Autodesk Inventor part; units mm, degrees
ref_plane "Work Plane1" through (60.325, 6.35, 63.5) normal (1, 0, 0) x (0, 0, -1)
ref_plane "Work Plane2" through (60.325, 6.35, -26.9875) normal (1, 0, 0) x (0, 0, -1)
ref_plane "YZ Plane" through (0, 0, 0) normal (1, 0, 0) x (0, 1, 0)
sketch "Sketch1" plane through (0, 0, 0) normal (0, 1, 0) x (-1, 0, 0)
  line L0 (0, -88.9) -> (0, 88.9)
  line L1 (-102.235, 0) -> (124.46, 0)
  line L2 (50.8, 44.45) -> (-50.8, 44.45)
  line L3 (-50.8, -44.45) -> (50.8, -44.45)
  line L4 (50.8, -44.45) -> (50.8, 44.45)
  line L5 (76.2, 63.5) -> (-69.85, 63.5)
  line L6 (-69.85, -63.5) -> (76.2, -63.5)
  line L7 (76.2, -63.5) -> (76.2, 63.5)
  line L8 (-50.8, 26.9875) -> (-69.85, 26.9875)
  line L9 (-69.85, -26.9875) -> (-50.8, -26.9875)
  line L10 (-50.8, 44.45) -> (-50.8, 26.9875)
  line L11 (-50.8, -26.9875) -> (-50.8, -44.45)
  line L12 (-69.85, 63.5) -> (-69.85, 26.9875)
  line L13 (-69.85, -26.9875) -> (-69.85, -63.5)
  line L14 (-53.975, 63.5) -> (-66.675, 63.5) construction
  line L15 (-66.675, 63.5) -> (-66.675, 26.9875) construction
  line L16 (-66.675, 26.9875) -> (-53.975, 26.9875) construction
  line L17 (-53.975, 26.9875) -> (-53.975, 63.5) construction
  line L18 (-53.975, -26.9875) -> (-66.675, -26.9875) construction
  line L19 (-66.675, -26.9875) -> (-66.675, -63.5) construction
  line L20 (-66.675, -63.5) -> (-53.975, -63.5) construction
  line L21 (-53.975, -63.5) -> (-53.975, -26.9875) construction
  line L22 (-60.325, 63.5) -> (-60.325, 26.9875) construction
  line L23 (-60.325, -26.9875) -> (-60.325, -63.5) construction
  line L24 (76.2, 22.225) -> (92.075, 22.225)
  line L25 (92.075, 22.225) -> (92.075, -22.225)
  line L26 (92.075, -22.225) -> (76.2, -22.225)
  line L27 (76.2, -22.225) -> (76.2, 22.225)
  point P0 (0, 0)
  dimension "d0" = 12.7
  dimension "d1" = 136.525
  dimension "d2" = 53.975
  dimension "d3" = 26.9875
  dimension "d4" = 101.6
  dimension "d5" = 19.05
  dimension "d6" = 3.175
  dimension "d7" = 50.8
  dimension "d8" = 88.9
  dimension "d9" = 44.45
  dimension "d10" = 19.05
  dimension "d11" = 19.05
  dimension "d24" = 25.4
  dimension "d25" = 44.45
  dimension "d26" = 22.225
  dimension "d27" = 41.275
extrude "Extrusion1" add sketch "Sketch1" along normal mid plane 12.7 contours L6 L13 L9 L11 L3 L0 | L0 L3 L4 L1 L7 L6 | L7 L1 L25 L26 | L2 L10 L8 L12 L5 L0 | L0 L5 L7 L1 L4 L2 | L7 L24 L25 L1
sketch "Sketch2" plane through (0, 6.35, 0) normal (0, 1, 0) x (1, 0, 0)
  line L0 (50.8, -44.45) -> (-50.8, -44.45)
  line L1 (-50.8, -44.45) -> (-50.8, 44.45)
  line L2 (-50.8, 44.45) -> (50.8, 44.45)
  line L3 (50.8, 44.45) -> (50.8, 26.9875)
  line L4 (50.8, 26.9875) -> (69.85, 26.9875)
  line L5 (69.85, 26.9875) -> (69.85, 63.5)
  line L6 (69.85, 63.5) -> (-76.2, 63.5)
  line L7 (-76.2, -22.225) -> (-76.2, -63.5)
  line L8 (-76.2, -63.5) -> (69.85, -63.5)
  line L9 (69.85, -63.5) -> (69.85, -26.9875)
  line L10 (69.85, -26.9875) -> (50.8, -26.9875)
  line L11 (50.8, -26.9875) -> (50.8, -44.45)
  line L12 (-76.2, -63.5) -> (69.85, -63.5)
  line L13 (53.975, -63.5) -> (66.675, -63.5)
  line L14 (66.675, -63.5) -> (66.675, -26.9875)
  line L15 (66.675, -26.9875) -> (53.975, -26.9875)
  line L16 (53.975, -26.9875) -> (53.975, -63.5)
  line L17 (50.8, 26.9875) -> (69.85, 26.9875)
  line L18 (69.85, 63.5) -> (-76.2, 63.5)
  line L19 (53.975, 26.9875) -> (66.675, 26.9875)
  line L20 (66.675, 26.9875) -> (66.675, 63.5)
  line L21 (66.675, 63.5) -> (53.975, 63.5)
  line L22 (53.975, 63.5) -> (53.975, 26.9875)
  line L23 (60.325, -63.5) -> (60.325, 99.2856) construction
  line L24 (102.235, 0) -> (-124.46, 0)
  line L25 (-76.2, 22.225) -> (-92.075, 22.225)
  line L26 (-92.075, 22.225) -> (-92.075, -22.225)
  line L27 (-92.075, -22.225) -> (-76.2, -22.225)
  line L28 (-76.2, 63.5) -> (-76.2, 22.225)
  point P0 (0, 0)
  dimension "d14" = 12.7
  dimension "d15" = 6.35
  dimension "d16" = 19.05
  dimension "d17" = 3.175
extrude "Extrusion2" cut sketch "Sketch2" against normal blind 4.7625 contours L10 L14 L8 L16 | L22 L6 L20 L4
sketch "Sketch3" plane through (0, 6.35, 0) normal (0, 1, 0) x (1, 0, 0)
  line L0 (-50.8, 12.4641) -> (-90.8, 12.4641)
  line L1 (102.235, 0) -> (-124.46, 0)
  line L2 (53.975, -63.5) -> (53.975, -26.9875)
  line L3 (53.975, -26.9875) -> (50.8, -26.9875)
  line L4 (50.8, -26.9875) -> (50.8, -44.45)
  line L5 (50.8, -44.45) -> (-50.8, -44.45)
  line L6 (-50.8, -44.45) -> (-50.8, 44.45)
  line L7 (-50.8, 44.45) -> (50.8, 44.45)
  line L8 (50.8, 44.45) -> (50.8, 26.9875)
  line L9 (50.8, 26.9875) -> (53.975, 26.9875)
  line L10 (53.975, 26.9875) -> (53.975, 63.5)
  line L11 (53.975, 63.5) -> (-76.2, 63.5)
  line L12 (-76.2, -22.225) -> (-76.2, -63.5)
  line L13 (-76.2, -63.5) -> (53.975, -63.5)
  line L14 (-76.2, 63.5) -> (-76.2, 22.225)
  line L15 (-76.2, 22.225) -> (-92.075, 22.225)
  line L16 (-92.075, 22.225) -> (-92.075, -22.225)
  line L17 (-92.075, -22.225) -> (-76.2, -22.225)
  point P0 (0, 0)
  point P1 (-87.5625, 16)
  point P2 (-55.5625, 16)
  point P3 (-55.5625, -16)
  point P4 (-87.5625, -16)
  dimension "d20" = 32
  dimension "d21" = 32
  dimension "d22" = 16
  dimension "d23" = 4.7625
hole "Hole1" at (-87.5625, 6.35, -16) at (-55.5625, 6.35, -16) at (-55.5625, 6.35, 16) at (-87.5625, 6.35, 16) direction (0, -1, 0) diameter 3.81 end through all counterbore diameter 7.1374 counterbore depth 3.5052
fillet "Fillet1" radius 6.35 6 edges at (-76.2, 0, 22.225) (-76.2, 0, -22.225) (-50.8, 0, -44.45) (-50.8, 0, 44.45) (50.8, 0, 44.45) (50.8, 0, -44.45)
chamfer "Chamfer1" distance 1.5875 angle 45 8 edges at (-92.075, 0, 22.225) (-92.075, 0, -22.225) (69.85, 0, 26.9875) (50.8, 0, 26.9875) (69.85, 0, 63.5) (69.85, 0, -26.9875) (69.85, 0, -63.5) (50.8, 0, -26.9875)
chamfer "Chamfer2" distance 6.35 angle 45 2 edges at (-76.2, 0, 63.5) (-76.2, 0, -63.5)
ref_plane "Work Plane1" through (60.325, 6.35, 63.5) normal (1, 0, 0) x (0, 0, -1)
ref_plane "Work Plane2" through (60.325, 6.35, -26.9875) normal (1, 0, 0) x (0, 0, -1)
sketch "Sketch4" plane through (0, 1.5875, 0) normal (0, 1, 0) x (1, 0, 0)
  line L0 (53.975, 63.5) -> (66.675, 63.5)
  line L1 (53.975, 26.9875) -> (53.975, 63.5)
  line L2 (66.675, 26.9875) -> (53.975, 26.9875)
  line L3 (66.675, 63.5) -> (66.675, 26.9875)
  line L4 (53.975, -26.9875) -> (66.675, -26.9875)
  line L5 (53.975, -63.5) -> (53.975, -26.9875)
  line L6 (66.675, -63.5) -> (53.975, -63.5)
  line L7 (66.675, -26.9875) -> (66.675, -63.5)
  point P0 (0, 0)
  point P1 (60.325, 42.8625)
  point P2 (60.325, -42.8625)
  dimension "d44" = 15.875
  dimension "d45" = 15.875
  dimension "d46" = 6.35
hole "Hole2" at (60.325, 1.5875, -42.8625) at (60.325, 1.5875, 42.8625) direction (0, -1, 0) diameter 3.302 end through all
chamfer "Chamfer3" distance 0.7937 angle 45 8 edges at (53.975, 3.9687, 63.5) (66.675, 3.9687, 63.5) (53.975, 3.9687, 26.9875) (66.675, 3.9687, 26.9875) (53.975, 3.9687, -26.9875) (66.675, 3.9687, -26.9875) (53.975, 3.9687, -63.5) (66.675, 3.9687, -63.5)
equation "\"d3\" = 0.5 * d2"
equation "\"d7\" = 0.5 * d4"
equation "\"d9\" = 0.5 * d8"
equation "\"d11\" = d10"
equation "\"d26\" = 0.5 * d25"
properties part number "Holder - headbars - L - LH" material "Stainless Steel"
Model file for the job. Use its own axes, mm. A direction names the side the tool comes from. Coordinates: 2 decimals unless noted, no trailing zeros. Order: outer loops, then holes, each group sorted by start corner. A loop starts at its lowest first (then second) coordinate and runs counter-clockwise, first axis right, second up. Notation, with made-up numbers: (49, 76.5) -> (60, 76.5) arc R14 cw to (60, 94.5) -> close; hole circle Ø9 at (10.25, -1.5). An arc over 180 degrees is marked (long way). Answer as a JSON object with one key per item and string values. Group by question number.
1) Flat gauge pins, fed straight in: pin 1 (6 mm diameter, centred on y = 2, z = 49.5, fed in from -X); pin 2 (6 mm diameter, centred on x = -87.56, z = -16, fed in from +Y); pin 3 (2.5 mm diameter, centred on x = -84.5, y = 1.5, fed in from +Z) (3 decimals). Where does each tip first touch, or does it go through?
2) Cut at D-D, the plane x = -74.5. Write the cut outline in (y, z), then the cut area to 3 significant figures.
3) Pull direction X, two halves, no side cores. Call faces 1 (the face through (-73.07, 0.09, -60.28)), 2 (the face through (68, 6.35, -45)), 3 (the face through (-1, 0, 44.45)): +X half, -X half, draft (parallel to the pull), parting line (faces both ways), or undercut.
4) Cut at A-A, the plane z = 16. Count the separate pieces of the cut face and the enclosed holes in it, then the cut area to 3 significant figures.
5) Cut at B-B, the plane x = 2. Write the cut outline in (y, z).
6) Drill centre lines: L1, parallel to X at y = -3.5, z = 16 (1 decimal); L2, parallel to X at y = 3.8, z = -16 (3 decimals); L3, parallel to Z at x = 57, y = -5.25. Where is each one in solid material? Low to high.
7) Which spindle directions (+Z, -Z, +X, -X, +Y, -Y) get a long thin tool onto all of the face, cutting with end or side? Do faces 4 (the face through (50.8, 0, 33)), 5 (the face through (-86, 2.845, -14)), 6 (the face through (66.675, 4, -45)), 7 (the face through (-76.2, 0, 43)), 8 (the face through (-87, 0, -22.225)). Say none if no direction does.
Check values:
{
 "1": {"pin 1": "stops at x = -76.2", "pin 2": "stops at y = 2.84", "pin 3": "stops at z = 22.225"},
 "2": {"outline": "(-6.35, -58.85) -> (6.35, -58.85) -> (6.35, 58.85) -> (-6.35, 58.85) -> close", "area": "1,490 mm²"},
 "3": {"face 1": "-X half", "face 2": "draft", "face 3": "undercut"},
 "4": {"separate pieces": "3", "enclosed holes": "0", "area": "404 mm²"},
 "5": {"outline": "(-6.35, -63.5) -> (6.35, -63.5) -> (6.35, -44.45) -> (-6.35, -44.45) -> close; (-6.35, 44.45) -> (6.35, 44.45) -> (6.35, 63.5) -> (-6.35, 63.5) -> close"},
 "6": {"L1": "x = -92.1 to -89.5, -85.7 to -57.5, -53.7 to -50.8", "L2": "x = -92.075 to -91.131, -83.994 to -59.131, -51.994 to -50.8", "L3": "z = -63.5 to -26.99, 26.99 to 63.5"},
 "7": {"face 4": "+Y, -Y", "face 5": "+Y", "face 6": "+Z, -Z, +Y", "face 7": "+Z, -X, +Y, -Y", "face 8": "-Z, -X, +Y, -Y"}
}
